from build123d import *

# Parameters (mm, degrees)
SKETCH1_R           = 22.5
BOSS_EXTRUDE1_DEPTH = 10
BOSS_EXTRUDE2_DEPTH = 20
SKETCH3_R           = 16.5
CUT_EXTRUDE2_DEPTH  = 5


with BuildPart() as part:
    # Sketch1 → Boss-Extrude1 (new body)
    with BuildSketch(Plane(origin=(0, 0, 0), x_dir=(1, 0, 0), z_dir=(0, 1, 0))):
        Circle(SKETCH1_R)
    extrude(amount=BOSS_EXTRUDE1_DEPTH)

    # Sketch2 → Boss-Extrude2 (add)
    with BuildSketch(Plane(origin=(0, 10, 0), x_dir=(1, 0, 0), z_dir=(0, 1, 0))):
        with BuildLine():
            Line((-29, 30), (29, 30))
            ThreePointArc((29, 30), (29.707106781, 29.707106781), (30, 29))
            Line((30, 29), (30, -29))
            ThreePointArc((30, -29), (29.707106781, -29.707106781), (29, -30))
            Line((29, -30), (-29, -30))
            ThreePointArc((-29, -30), (-29.707106781, -29.707106781), (-30, -29))
            Line((-30, -29), (-30, 29))
            ThreePointArc((-30, 29), (-29.707106781, 29.707106781), (-29, 30))
        make_face()
    extrude(amount=BOSS_EXTRUDE2_DEPTH)

    # Sketch3 → Cut-Extrude2 (cut)
    with BuildSketch(Plane.XZ):
        with BuildLine():
            ThreePointArc((-14.551420086, 2.778571429), (0, 11.5), (14.551420086, 2.778571429))
            Line((14.551420086, 2.778571429), (4.83856504, 20.948467447))
            ThreePointArc((4.83856504, 20.948467447), (0, 21.5), (-4.83856504, 20.948467447))
            Line((-4.83856504, 20.948467447), (-14.551420086, 2.778571429))
        make_face()
        with Locations((0, -5)):
            Circle(SKETCH3_R)
    extrude(amount=-CUT_EXTRUDE2_DEPTH, mode=Mode.SUBTRACT)


solid = part.part
Geometry check sheet. Reference: the model listing, model coordinates, mm. A direction names the side the tool comes from. Round coordinates to 2 decimals unless told otherwise and drop trailing zeros. Write each loop counter-clockwise with the first axis right and the second up, starting at its lowest first coordinate (ties: lowest second). Pieces come first, ordered by that corner, then holes. Notation, with made-up numbers: (44.5, 30.5) - (85.5, 30.5) arc R25 ccw to (85.5, 45.5) - close; hole circle Ø7 at (-17.5, 72). An arc over 180 degrees is marked (long way). One line per item, written item: value.
1. Depth check by flat-ended pin: pin 1 Ø4 at (x, y) = (3, 6) entering from -Z; pin 2 Ø20 at (x, z) = (0, -5) entering from -Y. Enter the tip coordinate at first touch or a pass-through.
The answers:
pin 1: stops at z = -22.48
pin 2: stops at y = 5
2. Mould release check, pull along Z, two halves, no side actions. Record for faces 1 (the face through (0, 20, 30)), 2 (the face through (10.382, 4.93, 19.961)), 3 (the face through (30, 20, 0)), 4 (the face through (0, 5, 0)): released by +Z, released by -Z, zero draft, split by the parting line, or undercut.
The answers:
face 1: released by +Z
face 2: split by the parting line
face 3: zero draft
face 4: undercut
3. Scan lines: L1, parallel to Y at x = 6, z = -24.5; L2, parallel to Y at x = -12, z = 4; L3, parallel to X at y = 2.8, z = -5. Record each from-to range of solid material in increasing order.
The answers:
L1: y = 10 to 30
L2: y = 5 to 30
L3: x = -21.94 to -16.5, 16.5 to 21.94
4. Cross-section at B-B on x = 0. Record the boundary of the cut face in (y, z).
The answers:
outline: (0, -22.5) - (10, -22.5) - (10, -30) - (30, -30) - (30, 30) - (10, 30) - (10, 22.5) - (0, 22.5) - (0, 21.5) - (5, 21.5) - (5, -21.5) - (0, -21.5) - close
5. Set-up check for faces 5 (the face through (-30, 20, 0)), 6 (the face through (14, 10, -20)): record each of +Z, -Z, +X, -X, +Y, -Y from which the full face is reachable in a straight line by a thin tool's end or side.
The answers:
face 5: +Z, -Z, -X, +Y, -Y
face 6: -Y
6. Cross-section at A-A on z = -3. Record the boundary of the cut face in (x, y), and give its area (3 significant figures).
The answers:
outline: (-30, 10) - (-22.3, 10) - (-22.3, 0) - (-16.38, 0) - (-16.38, 5) - (16.38, 5) - (16.38, 0) - (22.3, 0) - (22.3, 10) - (30, 10) - (30, 30) - (-30, 30) - close
area: 1,480 mm^2
7. Cross-section at C-C on z = -26. Record the boundary of the cut face in (x, y), and give its area (3 significant figures).
The answers:
outline: (-30, 10) - (30, 10) - (30, 30) - (-30, 30) - close
area: 1,200 mm^2
